Geometry: see drawing. Coordinates: mm, zero at the bounding-box minimum. A direction names the side the tool comes from. Give positions to 0.01 mm unless a question says otherwise; leave off trailing zeros. Loops run counter-clockwise (first coordinate to the right, second up) from the corner with the lowest first, then second, coordinate; pieces in that order, holes last. Notation, with made-up numbers: M 62.5,-3 L 87.5,-3 A13 cw 87.5,17 Z; hole C 32.5,26 d7. An arc over 180 degrees is marked long. Put each result on its own line as item: value.
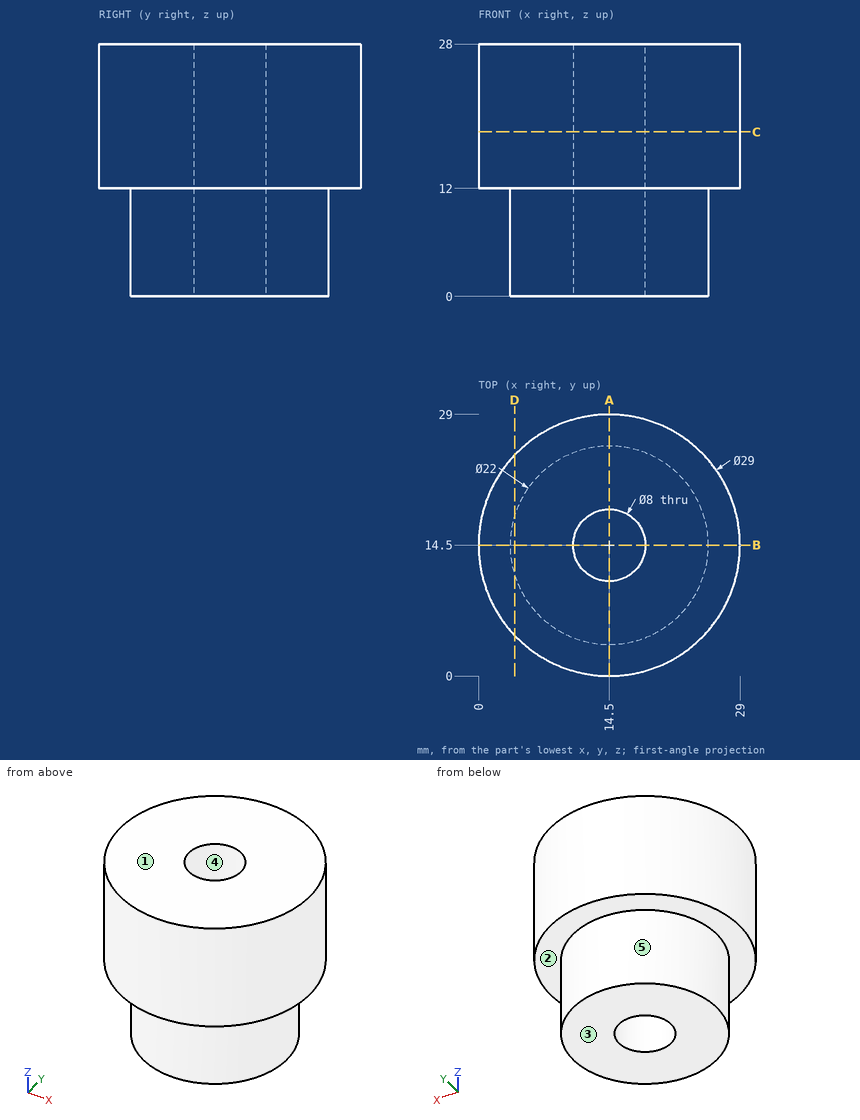
1. Contact query for flat-ended pins moving along their axis: P1, Ø12, axis at x = 9.5, z = 15, coming from the -Y side; P2, Ø1.5, axis at y = 18.5, z = 14, coming from the -X side; P3, Ø4, axis at x = 20.5, z = 11, coming from the +Y side; P4, Ø2, axis at y = 4, z = 7.5, coming from the -X side. Output: stop coordinate, or through.
Found:
P1: y = 0
P2: x = 0.37
P3: y = 28.36
P4: x = 8.95
2. Section query A-A (x = 14.5). Output: boundary loops of the cut face in (y, z), plus the area to 3 significant figures.
Found:
outline: M 0,12 L 3.5,12 L 3.5,0 L 10.5,0 L 10.5,28 L 0,28 Z; M 18.5,0 L 25.5,0 L 25.5,12 L 29,12 L 29,28 L 18.5,28 Z
area: 504 mm^2
3. Section query D-D (x = 4). Output: boundary loops of the cut face in (y, z).
Found:
outline: M 4.5,12 L 11.22,12 L 11.22,0 L 17.78,0 L 17.78,12 L 24.5,12 L 24.5,28 L 4.5,28 Z
4. Draft query along X for the marked faces 3, 4 and 5. Return one class per face: pulls with the +X half, pulls with the -X half, needs draft (parallel to the pull), parting line crosses it, or undercut.
Found:
face 3: needs draft
face 4: undercut
face 5: parting line crosses it
5. Access query for the marked faces 1 and 2. Directions: +Z, -Z, +X, -X, +Y, -Y. A direction counts if a zero-diameter tool reaches every point of the face in a straight line with its end or side. Return the directions, or none.
Found:
face 1: +Z, +X, -X, +Y, -Y
face 2: -Z
6. Material intervals for line 1 (Y direction, x = 14.5, z = 13); line 2 (Z direction, x = 27, y = 17); line 3 (X direction, y = 12, z = 20.5), sorted ascending. Write a range as from..to.
Found:
line 1: 0..10.5, 18.5..29
line 2: 12..28
line 3: 0.22..11.38, 17.62..28.78
7. Section query C-C (z = 18.25). Output: boundary loops of the cut face in (x, y).
Found:
outline: C 14.5,14.5 d29; hole C 14.5,14.5 d8
